Can you work these out from the model? Positions are in its coordinate system, mm. Give positions to 0.01 mm unless a question says otherwise; leave off trailing zeros. Order: outer loops, then holes, each group sorted by start corner. A loop starts at its lowest first (then second) coordinate and runs counter-clockwise, first axis right, second up. Notation, with made-up numbers: (78.25, 8) - (113.25, 8) arc R9 ccw to (113.25, 22) - close; hole circle Ø8 at (-40, 47). An arc over 180 degrees is marked (long way). Use one line per item in the form item = value. Start each with the question number.
1) For pin 1 (1.8 mm diameter, centred on x = -3.92, y = -14.29, fed in from -Z); pin 2 (2 mm diameter, centred on x = -4, z = 2.5, fed in from +Y), each with a flat end and sliding along its axis, tell me the tip position at first contact or that it passes through.
2) Suppose I cut it at D-D, the plane y = 21.5. Write out the boundary of the cut face in (x, z), and give its area (3 significant figures).
3) Suppose I cut it at B-B, the plane z = 2.25. Write out the boundary of the cut face in (x, y) (3 decimals).
4) Please list where these lines run through material, in increasing order: probe 1 along Y at (x, z) = (15.5, 0.9); probe 2 along Y at (x, z) = (-4.5, 2.95); probe 3 along X at (y, z) = (-14.5, 3.15).
5) Suppose I cut it at A-A, the plane x = -16.5. Write out the boundary of the cut face in (y, z).
6) We'd pull the mould along Y, two halves only. Please class faces 1 (the flat face through (-10, 0, 4)), 2 (the flat face through (-12.694, 9.624, 1.972)), 3 (the cylindrical face through (-34.53, -14.86, 1.97)), 4 (the flat face through (10.3, 2.85, 1.97)): released by +Y, released by -Y, zero draft, split by the parting line, or undercut.
7) Suppose I cut it at C-C, the plane x = 15. Write out the boundary of the cut face in (y, z), and give its area (3 significant figures).
```python
from build123d import *

# Parameters (mm, degrees)
SKETCH_1_R      = 1.5
SKETCH_1_R_2    = 1.55
EXTRUDE_1_DEPTH = 4


with BuildPart() as part:
    # 草图1 → 凸台-拉伸1 (new body)
    with BuildSketch(Plane.XY):
        with BuildLine():
            Line((12.826389613, 29.00362922), (-38.939235387, -10.306930028))
            ThreePointArc((-38.939235387, -10.306930028), (-40.654009304, -15.884229397), (-35.915346214, -19.288901182))
            Line((-35.915346214, -19.288901182), (-3.915346214, -19.288901182))
            ThreePointArc((-3.915346214, -19.288901182), (-1.291462523, -18.545100704), (0.551762792, -16.534994932))
            Line((0.551762792, -16.534994932), (20.317387792, 22.775564316))
            ThreePointArc((20.317387792, 22.775564316), (19.046826765, 28.866405264), (12.826389613, 29.00362922))
        make_face()
        with Locations((15.850278786, 25.021658066)):
            Circle(SKETCH_1_R, mode=Mode.SUBTRACT)
        with Locations((-3.915346214, -14.288901182)):
            Circle(SKETCH_1_R, mode=Mode.SUBTRACT)
        with Locations((-35.915346214, -14.288901182)):
            Circle(SKETCH_1_R, mode=Mode.SUBTRACT)
        with Locations((-19.987461598, -2.19334449)):
            Circle(SKETCH_1_R, mode=Mode.SUBTRACT)
        with Locations((-15.915346214, -15.288901182)):
            Circle(SKETCH_1_R_2, mode=Mode.SUBTRACT)
    extrude(amount=EXTRUDE_1_DEPTH)


solid = part.part
```
Result sheet:
q1.pin_1 = through
q1.pin_2 = 16.99
q2.outline = (2.95, 0) - (19.68, 0) - (19.68, 4) - (2.95, 4) - close
q2.area = 66.9 mm²
q3.outline = (-38.939, -10.307) arc R5 ccw to (-35.915, -19.289) - (-3.915, -19.289) arc R5 ccw to (0.552, -16.535) - (20.317, 22.776) arc R5 ccw to (12.826, 29.004) - close; hole circle Ø3 at (-35.915, -14.289); hole circle Ø3 at (-19.987, -2.193); hole circle Ø3.1 at (-15.915, -15.289); hole circle Ø3 at (-3.915, -14.289); hole circle Ø3 at (15.85, 25.022)
q4.probe_1 = 13.19 to 23.56, 26.48 to 30.01
q4.probe_2 = -19.29 to -15.67, -12.91 to 15.85
q4.probe_3 = -40.91 to -37.4, -34.43 to -17.25, -14.58 to -5.4, -2.43 to 1.57
q5.outline = (-19.29, 0) - (-16.72, 0) - (-16.72, 4) - (-19.29, 4) - close; (-13.85, 0) - (6.73, 0) - (6.73, 4) - (-13.85, 4) - close
q6.face_1 = zero draft
q6.face_2 = released by +Y
q6.face_3 = undercut
q6.face_4 = released by -Y
q7.outline = (12.2, 0) - (23.79, 0) - (23.79, 4) - (12.2, 4) - close; (26.26, 0) - (29.95, 0) - (29.95, 4) - (26.26, 4) - close
q7.area = 61.1 mm²
